Can you work these out from the model? Positions are in its coordinate system, mm. Face numbers are marked on the shaded views. A direction names the side the tool comes from. Coordinates: 2 decimals unless noted, no trailing zeros. Order: outer loops, then holes, each group sorted by start corner. A loop starts at its lowest first (then second) coordinate and runs counter-clockwise, first axis right, second up.
```python
from build123d import *

# Parameters (mm, degrees)
SKETCH_1_R               = 6.325
EXTRUDE_1_DEPTH          = 15
SKETCH_2_W               = 28.5
SKETCH_2_H               = 18
EXTRUDE_2_DEPTH          = 3
EXTRUDE_START            = 14.25
SKETCH_4_R               = 1.65
EXTRUDE_3_DEPTH          = 7
EXTRUDE_START_2          = -14.25
SKETCH_4_2_R             = 1.65
EXTRUDE_4_DEPTH          = 7
EXTRUDE_5_DEPTH          = 7
SKETCH_7_R               = 1.8
CUT_EXTRUDE_1_DEPTH      = 19
CUT_EXTRUDE_3_DEPTH      = 1
CUT_EXTRUDE_3_DEPTH_BACK = 29.5
SKETCH_10_R              = 12.25
SKETCH_10_R_2            = 9.25
EXTRUDE_6_DEPTH          = 15
EXTRUDE_7_DEPTH          = 3
CUT_EXTRUDE_4_DEPTH      = 15.25
CUT_EXTRUDE_4_DEPTH_BACK = 15.25
SKETCH_13_W              = 7.383863518
SKETCH_13_H              = 7
CUT_EXTRUDE_5_DEPTH      = 12
CUT_EXTRUDE_6_DEPTH      = 1.0000001
CUT_EXTRUDE_6_DEPTH_BACK = 61
CHAMFER_3_SIZE           = 1
CHAMFER_3_SIZE2          = 5.67128182


with BuildPart() as part:
    # ｽｹｯﾁ1 → ﾎﾞｽ - 押し出し1 (new body)
    with BuildSketch(Plane.XY):
        Circle(SKETCH_1_R)
    extrude(amount=EXTRUDE_1_DEPTH)

    # ｽｹｯﾁ2 → ﾎﾞｽ - 押し出し2 (add)
    with BuildSketch(Plane.XY.offset(15)):
        Rectangle(SKETCH_2_W, SKETCH_2_H)
    extrude(amount=EXTRUDE_2_DEPTH)

    # ｽｹｯﾁ4 → ﾎﾞｽ - 押し出し3 (add)
    with BuildSketch(Plane(origin=(0, 0, 0), x_dir=(0, 0, -1), z_dir=(1, 0, 0)).offset(EXTRUDE_START)):
        with BuildLine():
            Line((-54.074074074, 13.913518208), (-28, 9))
            Line((-28, 9), (-18, 9))
            Line((-18, 9), (-18, -9))
            Line((-18, -9), (-56.624751337, 4.271344473))
            ThreePointArc((-56.624751337, 4.271344473), (-59.833732287, 10.278683768), (-54.074074074, 13.913518208))
        make_face()
        with Locations((-55, 9)):
            Circle(SKETCH_4_R, mode=Mode.SUBTRACT)
    extrude(amount=-EXTRUDE_3_DEPTH)

    # ｽｹｯﾁ4<2> → ﾎﾞｽ - 押し出し4 (add)
    with BuildSketch(Plane(origin=(0, 0, 0), x_dir=(0, 0, -1), z_dir=(1, 0, 0)).offset(EXTRUDE_START_2)):
        with BuildLine():
            Line((-54.074074074, 13.913518208), (-28, 9))
            Line((-28, 9), (-18, 9))
            Line((-18, 9), (-18, -9))
            Line((-18, -9), (-56.624751337, 4.271344473))
            ThreePointArc((-56.624751337, 4.271344473), (-59.833732287, 10.278683768), (-54.074074074, 13.913518208))
        make_face()
        with Locations((-55, 9)):
            Circle(SKETCH_4_2_R, mode=Mode.SUBTRACT)
    extrude(amount=EXTRUDE_4_DEPTH)

    # ｽｹｯﾁ5 → ﾎﾞｽ - 押し出し5 (add)
    with BuildSketch(Plane.ZY.offset(14.25)):
        with BuildLine():
            Line((18, -9), (33.823085464, -9))
            Line((33.823085464, -9), (57.5, 4.669872981))
            ThreePointArc((57.5, 4.669872981), (57.071979643, 4.44951647), (56.624751337, 4.271344473))
            Line((56.624751337, 4.271344473), (18, -9))
        make_face()
    extrude_5 = extrude(amount=-EXTRUDE_5_DEPTH)

    # ﾐﾗｰ1: ﾎﾞｽ - 押し出し5 across plane
    add(extrude_5.mirror(Plane(origin=(0, 0, 0), x_dir=(0, 0, 1), z_dir=(1, 0, 0))))

    # ｽｹｯﾁ7 → ｶｯﾄ - 押し出し1 (cut, through all)
    with BuildSketch(Plane(origin=(0, 9, 0), x_dir=(1, 0, 0), z_dir=(0, 1, 0))):
        with Locations((10.75, -23)):
            Circle(SKETCH_7_R)
        with Locations((-10.75, -23)):
            Circle(SKETCH_7_R)
    extrude(amount=-CUT_EXTRUDE_1_DEPTH, mode=Mode.SUBTRACT)

    # ｽｹｯﾁ9 → ｶｯﾄ - 押し出し3 (cut, two sides)
    with BuildSketch(Plane(origin=(14.25, 0, 0), x_dir=(0, 0, -1), z_dir=(1, 0, 0))) as cut_extrude_3_sk:
        Polygon((-15, 127.875853754), (-15, 12.993387334), (-15, -12.927364159), (-15, -127.809830579), (214.76493284, -127.809830579), (214.76493284, 127.875853754), align=None)
    extrude(amount=CUT_EXTRUDE_3_DEPTH, mode=Mode.SUBTRACT)
    extrude(cut_extrude_3_sk.sketch, amount=-CUT_EXTRUDE_3_DEPTH_BACK, mode=Mode.SUBTRACT)

    # ｽｹｯﾁ10 → ﾎﾞｽ - 押し出し6 (add)
    with BuildSketch(Plane(origin=(0, 0, 15), x_dir=(-1, 0, 0), z_dir=(0, 0, -1))):
        Circle(SKETCH_10_R)
        Circle(SKETCH_10_R_2, mode=Mode.SUBTRACT)
    extrude(amount=EXTRUDE_6_DEPTH)

    # ｽｹｯﾁ11 → ﾎﾞｽ - 押し出し7 (add)
    with BuildSketch(Plane(origin=(0, 0, 15), x_dir=(-1, 0, 0), z_dir=(0, 0, -1))):
        with BuildLine():
            Line((8.310385069, -9), (14.25, -9))
            Line((14.25, -9), (14.25, 9))
            Line((14.25, 9), (8.310385069, 9))
            ThreePointArc((8.310385069, 9), (12.25, 0), (8.310385069, -9))
        make_face()
        with BuildLine():
            Line((-8.310385069, 9), (-14.25, 9))
            Line((-14.25, 9), (-14.25, -9))
            Line((-14.25, -9), (-8.310385069, -9))
            ThreePointArc((-8.310385069, -9), (-12.25, 0), (-8.310385069, 9))
        make_face()
    extrude(amount=EXTRUDE_7_DEPTH)

    # ｽｹｯﾁ12 → ｶｯﾄ - 押し出し4 (cut, two sides)
    with BuildSketch(Plane(origin=(0, 0, 0), x_dir=(0, 0, -1), z_dir=(1, 0, 0))) as cut_extrude_4_sk:
        with BuildLine():
            Line((-9.405255888, 0), (-8.928941916, 0.825))
            ThreePointArc((-8.928941916, 0.825), (-5.85, 0), (-8.928941916, -0.825))
            Line((-8.928941916, -0.825), (-9.405255888, 0))
        make_face()
    extrude(amount=CUT_EXTRUDE_4_DEPTH, mode=Mode.SUBTRACT)
    extrude(cut_extrude_4_sk.sketch, amount=-CUT_EXTRUDE_4_DEPTH_BACK, mode=Mode.SUBTRACT)

    # ｽｹｯﾁ13 → ｶｯﾄ - 押し出し5 (cut)
    with BuildSketch(Plane(origin=(0, 0, 0), x_dir=(-1, 0, 0), z_dir=(0, 0, -1))):
        with Locations((15.431288641, 0)):
            Rectangle(SKETCH_13_W, SKETCH_13_H)
        with Locations((-15.431288641, 0)):
            Rectangle(SKETCH_13_W, SKETCH_13_H)
    extrude(amount=-CUT_EXTRUDE_5_DEPTH, mode=Mode.SUBTRACT)

    # ｽｹｯﾁ14 → ｶｯﾄ - 押し出し6 (cut, two sides)
    with BuildSketch(Plane(origin=(0, 0, 0), x_dir=(-1, 0, 0), z_dir=(0, 0, -1))) as cut_extrude_6_sk:
        Polygon((76.843424889, -11.578536177), (4, -11.578536177), (-4, -11.578536177), (-76.843424889, -11.578536177), (-76.843424889, -157.265385955), (76.843424889, -157.265385955), align=None)
    extrude(amount=CUT_EXTRUDE_6_DEPTH, mode=Mode.SUBTRACT)
    extrude(cut_extrude_6_sk.sketch, amount=-CUT_EXTRUDE_6_DEPTH_BACK, mode=Mode.SUBTRACT)

    # 面取り3
    chamfer_3_edges = [part.edges().sort_by_distance(p)[0] for p in [
        (0, -11.578536177, 0),
    ]]
    chamfer_3_side = [part.faces().sort_by_distance(p)[0] for p in [
        (-11.404834964, 0, 0),
    ]]
    chamfer(chamfer_3_edges, length=CHAMFER_3_SIZE, length2=CHAMFER_3_SIZE2, reference=chamfer_3_side[0])


solid = part.part
```
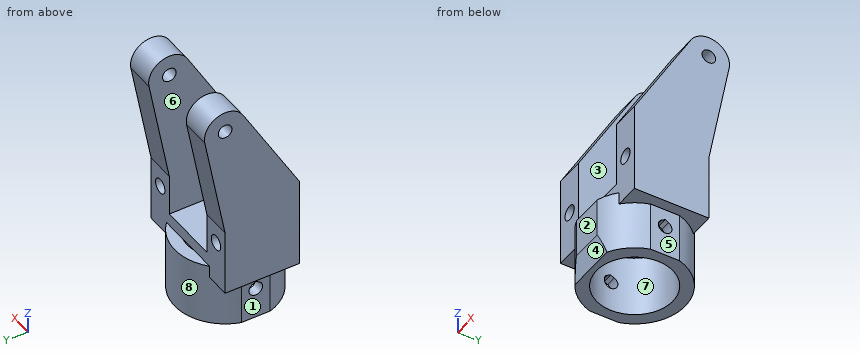
1. Imagine slicing it at A-A on z = 26. Please give me the cut outline in (x, y), then the cut area to 3 significant figures.
Completed:
outline: (-14.25, -9) - (-7.25, -9) - (-7.25, 9) - (-14.25, 9) - close; (7.25, -9) - (14.25, -9) - (14.25, 9) - (7.25, 9) - close
area: 252 mm2
2. Please list where these lines run through material, in increasing order: probe 1 along X at (y, z) = (4, 23); probe 2 along Y at (x, z) = (0, 9.25); probe 3 along X at (y, z) = (-0.5, 30).
Completed:
probe 1: x = -14.25 to -12.55, -8.95 to -7.25, 7.25 to 8.95, 12.55 to 14.25
probe 2: y = -11.58 to -9.25, 9.25 to 12.25
probe 3: x = -14.25 to -7.25, 7.25 to 14.25
3. On a 3-axis mill with a long thin cutter (end or side, diameter ignored), from which of +Z, -Z, +X, -X, +Y, -Y can I reach the whole of each face in a straight line? I mean the marked faces 4, 5, 6, 7 and 8. Say none if no direction works.
Completed:
face 4: -Z, +X, -X, -Y
face 5: -Z, +X, +Y, -Y
face 6: +Z, +Y, -Y
face 7: -Z
face 8: -Z, +Y
4. Imagine slicing it at B-B on x = 0. Please give me the cut outline in (y, z), then the cut area to 3 significant figures.
Completed:
outline: (-11.58, 5.67) - (-10.58, 0) - (-9.25, 0) - (-9.25, 15) - (-11.58, 15) - close; (-9, 15) - (9, 15) - (9, 18) - (-9, 18) - close; (9.25, 0) - (12.25, 0) - (12.25, 15) - (9.25, 15) - close
area: 131 mm2
5. Thinking about a two-plate mould opening in X: for the marked faces 1, 2 and 3, which applies, pulls with the +X half, pulls with the -X half, needs draft (parallel to the pull), parting line crosses it, or undercut?
Completed:
face 1: pulls with the -X half
face 2: needs draft
face 3: undercut
6. Imagine slicing it at D-D on x = -10.75. Please give me the cut outline in (y, z) (3 decimals).
Completed:
outline: (-9, 12) - (-5.874, 12) - (-5.874, 0) - (5.874, 0) - (5.874, 12) - (9, 12) - (9, 21.2) - (-9, 21.2) - close; (-9, 24.8) - (9, 24.8) - (9, 28) - (13.914, 54.074) arc R5 ccw to (4.67, 57.5) - (-9, 33.823) - close; hole (-0.825, 8.929) arc R1.65 ccw (long way) to (0.825, 8.929) - (0, 9.405) - close; hole circle Ø3.3 at (9, 55)
7. Imagine slicing it at C-C on z = 55. Please give me the cut outline in (x, y).
Completed:
outline: (-14.25, 3.23) - (-7.25, 3.23) - (-7.25, 7.35) - (-14.25, 7.35) - close; (-14.25, 10.65) - (-7.25, 10.65) - (-7.25, 14) - (-14.25, 14) - close; (7.25, 3.23) - (14.25, 3.23) - (14.25, 7.35) - (7.25, 7.35) - close; (7.25, 10.65) - (14.25, 10.65) - (14.25, 14) - (7.25, 14) - close
8. I'm going to push flat-ended pins straight in: pin 1 (6 mm diameter, centred on x = 10.75, z = 23, fed in from +Y); pin 2 (3.5 mm diameter, centred on y = -1.5, z = 7.5, fed in from +X); pin 3 (4.5 mm diameter, centred on x = -3, y = 4, fed in from +Z); pin 4 (5 mm diameter, centred on x = -0.5, z = 22, fed in from +Y). Where does each tip first touch, or does it pass through?
Completed:
pin 1: stops at y = 9
pin 2: stops at x = 11.74
pin 3: stops at z = 18
pin 4: passes through
